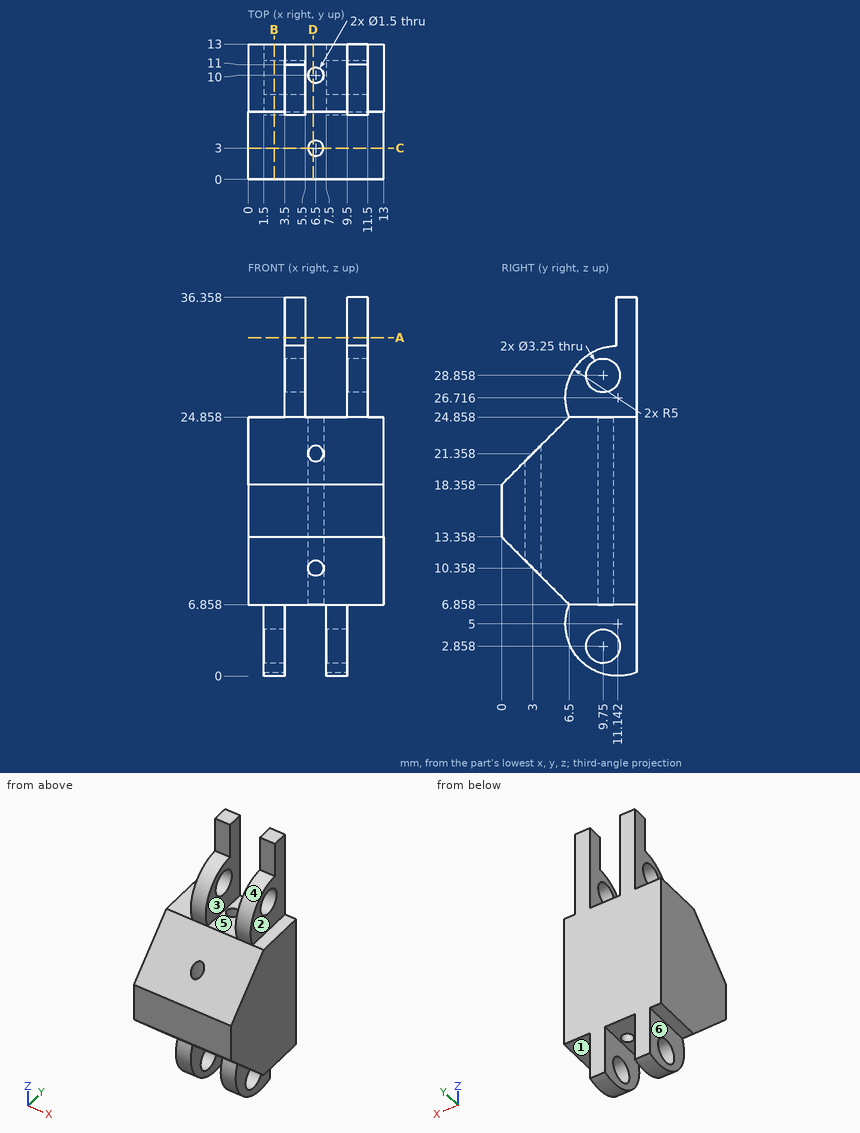
For this review, use the dimensioned drawing (mm, ordinates from the lowest corner) and the shaded views. A direction names the side the tool comes from. Give positions to 0.01 mm unless a question says otherwise; leave off trailing zeros. Loops run counter-clockwise (first coordinate to the right, second up) from the corner with the lowest first, then second, coordinate; pieces in that order, holes last. Notation, with made-up numbers: (-34.75, 81) -> (2.25, 81) arc R15 cw to (2.25, 97) -> close; hole circle Ø9 at (85.5, -19.75). An arc over 180 degrees is marked (long way). Use CSV: the item, a comma, the result in double quotes.
1. Consider section A-A, the plane z = 32.5. Write out the cut boundary in (x, y).
Result:
outline,"(3.5, 11) -> (5.5, 11) -> (5.5, 13) -> (3.5, 13) -> close; (9.5, 11) -> (11.5, 11) -> (11.5, 13) -> (9.5, 13) -> close"
2. The part is to be moulded in two halves that separate along X. For the marked faces 4, 5 and 6, say which applies: +X half, -X half, draft (parallel to the pull), parting line (faces both ways), or undercut.
Result:
face 4,"draft"
face 5,"undercut"
face 6,"-X half"
3. To check wall thickness, follow probe 1 along X at (y, z) = (8.25, 28); probe 2 along Y at (x, z) = (6.5, 19); probe 3 along X at (y, z) = (10, 6). State the ranges of each line that lie inside material, in increasing order. Write a range as from..to.
Result:
probe 1,"x = 3.5..5.5, 9.5..11.5"
probe 2,"y = 0.64..2.25, 3.75..9.25, 10.75..13"
probe 3,"x = 1.5..3.5, 7.5..9.5"
4. Consider section C-C, the plane y = 3. Write out the cut boundary in (x, z), then the cut area to 4 significant figures.
Result:
outline,"(0, 10.36) -> (5.75, 10.36) -> (5.75, 21.36) -> (0, 21.36) -> close; (7.25, 10.36) -> (13, 10.36) -> (13, 21.36) -> (7.25, 21.36) -> close"
area,"126.5 mm²"
5. Consider section D-D, the plane x = 6.25. Write out the cut boundary in (y, z) (1 decimal), then the cut area to 3 significant figures.
Result:
outline,"(0, 13.4) -> (2.3, 11.1) -> (2.3, 20.7) -> (0, 18.4) -> close; (3.7, 9.7) -> (6.5, 6.9) -> (9.3, 6.9) -> (9.3, 24.9) -> (6.5, 24.9) -> (3.7, 22.1) -> close; (10.7, 6.9) -> (13, 6.9) -> (13, 24.9) -> (10.7, 24.9) -> close"
area,"151 mm²"
6. Consider section B-B, the plane x = 2.5. Write out the cut boundary in (y, z) (3 decimals), then the cut area to 3 significant figures.
Result:
outline,"(0, 13.358) -> (6.5, 6.858) arc R5 ccw to (13, 0.358) -> (13, 24.858) -> (6.5, 24.858) -> (0, 18.358) -> close; hole circle Ø3.25 at (9.75, 2.858)"
area,"225 mm²"
7. For P1, Ø4, axis at y = 9.75, z = 2.86, coming from the +X side; P2, Ø4, axis at x = 10.5, y = 9.5, coming from the -Z side; P3, Ø7.5, axis at y = 9.5, z = 30, coming from the -X side; P4, Ø1, axis at x = 10, z = 34, coming from the -Y side, all flat-tipped, find the tip position at first contact; note any pin that passes through.
Result:
P1,"stops at x = 9.5"
P2,"stops at z = 0"
P3,"stops at x = 3.5"
P4,"stops at y = 11"
8. Machinability: for the marked faces 1, 2 and 3, which of the approach directions +Z, -Z, +X, -X, +Y, -Y give a long, thin tool a straight path to every point of the face, cutting with its end or side? Answer none if there is none.
Result:
face 1,"-Z, +X, +Y, -Y"
face 2,"+Z, +X, +Y, -Y"
face 3,"+Z, +Y, -Y"
